Model file for the job. Use its own axes, mm. Give positions to 0.01 mm unless a question says otherwise; leave off trailing zeros. Write each loop counter-clockwise with the first axis right and the second up, starting at its lowest first coordinate (ties: lowest second). Pieces come first, ordered by that corner, then holes. Notation, with made-up numbers: (53.25, 15.25) - (98.25, 15.25) arc R26 ccw to (98.25, 29.25) - close; hole circle Ø11 at (74, -7.5). An arc over 180 degrees is marked (long way). Use a Markdown table: item, result. Add a question column.
```python
from build123d import *

# Parameters (mm, degrees)
SKETCH1_R           = 2.5
BOSS_EXTRUDE1_DEPTH = 10
FILLET1_R           = 20
FILLET2_R           = 2


with BuildPart() as part:
    # Sketch1 → Boss-Extrude1 (new body)
    with BuildSketch(Plane(origin=(0, 0, 0), x_dir=(1, 0, 0), z_dir=(0, 1, 0))):
        with BuildLine():
            Line((0, 0), (0, 125))
            Line((0, 125), (-12.5, 155))
            Line((-12.5, 155), (-25, 125))
            Line((-25, 125), (-38.474856438, 113.744856999))
            ThreePointArc((-38.474856438, 113.744856999), (-43.483141428, 102.313155182), (-37.378629761, 91.427308304))
            Line((-37.378629761, 91.427308304), (-25, 83))
            Line((-25, 83), (-25, 25))
            Line((-25, 25), (-35, 25))
            Line((-35, 25), (-35, 73))
            ThreePointArc((-35, 73), (-37.928932188, 80.071067812), (-45, 83))
            Line((-45, 83), (-45, 58))
            ThreePointArc((-45, 58), (-57.043096437, 48.210936871), (-64.16515139, 62))
            Line((-64.16515139, 62), (-55, 83))
            Line((-55, 83), (-55, 125))
            Line((-55, 125), (-67.5, 155))
            Line((-67.5, 155), (-80, 125))
            Line((-80, 125), (-93.474856438, 113.744856999))
            ThreePointArc((-93.474856438, 113.744856999), (-98.483141428, 102.313155182), (-92.378629761, 91.427308304))
            Line((-92.378629761, 91.427308304), (-80, 83))
            Line((-80, 83), (-80, 25))
            Line((-80, 25), (-90, 25))
            Line((-90, 25), (-90, 73))
            ThreePointArc((-90, 73), (-92.928932188, 80.071067812), (-100, 83))
            Line((-100, 83), (-100, 58))
            ThreePointArc((-100, 58), (-112.043096437, 48.210936871), (-119.16515139, 62))
            Line((-119.16515139, 62), (-110, 83))
            Line((-110, 83), (-110, 125))
            Line((-110, 125), (-122.5, 155))
            Line((-122.5, 155), (-135, 125))
            Line((-135, 125), (-148.474856438, 113.744856999))
            ThreePointArc((-148.474856438, 113.744856999), (-153.483141428, 102.313155182), (-147.378629761, 91.427308304))
            Line((-147.378629761, 91.427308304), (-135, 83))
            Line((-135, 83), (-135, 25))
            Line((-135, 25), (-145, 25))
            Line((-145, 25), (-145, 73))
            ThreePointArc((-145, 73), (-147.928932188, 80.071067812), (-155, 83))
            Line((-155, 83), (-155, 58))
            ThreePointArc((-155, 58), (-167.043096437, 48.210936871), (-174.16515139, 62))
            Line((-174.16515139, 62), (-165, 83))
            Line((-165, 83), (-165, 125))
            Line((-165, 125), (-177.5, 155))
            Line((-177.5, 155), (-190, 125))
            Line((-190, 125), (-203.474856438, 113.744856999))
            ThreePointArc((-203.474856438, 113.744856999), (-208.483141428, 102.313155182), (-202.378629761, 91.427308304))
            Line((-202.378629761, 91.427308304), (-190, 83))
            Line((-190, 83), (-190, 25))
            Line((-190, 25), (-200, 25))
            Line((-200, 25), (-200, 73))
            ThreePointArc((-200, 73), (-202.928932188, 80.071067812), (-210, 83))
            Line((-210, 83), (-210, 58))
            ThreePointArc((-210, 58), (-222.043096437, 48.210936871), (-229.16515139, 62))
            Line((-229.16515139, 62), (-220, 83))
            Line((-220, 83), (-220, 125))
            Line((-220, 125), (-232.5, 155))
            Line((-232.5, 155), (-245, 125))
            Line((-245, 125), (-258.474856438, 113.744856999))
            ThreePointArc((-258.474856438, 113.744856999), (-263.483141428, 102.313155182), (-257.378629761, 91.427308304))
            Line((-257.378629761, 91.427308304), (-245, 83))
            Line((-245, 83), (-245, 25))
            Line((-245, 25), (-255, 25))
            Line((-255, 25), (-255, 73))
            ThreePointArc((-255, 73), (-257.928932188, 80.071067812), (-265, 83))
            Line((-265, 83), (-265, 58))
            ThreePointArc((-265, 58), (-277.043096437, 48.210936871), (-284.16515139, 62))
            Line((-284.16515139, 62), (-275, 83))
            Line((-275, 83), (-275, 125))
            Line((-275, 125), (-287.5, 155))
            Line((-287.5, 155), (-300, 125))
            Line((-300, 125), (-300, 0))
            Line((-300, 0), (0, 0))
        make_face()
        with Locations(Location((-12.5, 125, 0), (0, 0, 270))):
            Circle(SKETCH1_R, mode=Mode.SUBTRACT)
        with Locations(Location((-64, 89, 0), (0, 0, 270))):
            Circle(SKETCH1_R, mode=Mode.SUBTRACT)
        with Locations(Location((-67.5, 125, 0), (0, 0, 270))):
            Circle(SKETCH1_R, mode=Mode.SUBTRACT)
        with Locations(Location((-119, 89, 0), (0, 0, 270))):
            Circle(SKETCH1_R, mode=Mode.SUBTRACT)
        with Locations(Location((-122.5, 125, 0), (0, 0, 270))):
            Circle(SKETCH1_R, mode=Mode.SUBTRACT)
        with Locations(Location((-174, 89, 0), (0, 0, 270))):
            Circle(SKETCH1_R, mode=Mode.SUBTRACT)
        with Locations(Location((-177.5, 125, 0), (0, 0, 270))):
            Circle(SKETCH1_R, mode=Mode.SUBTRACT)
        with Locations(Location((-229, 89, 0), (0, 0, 270))):
            Circle(SKETCH1_R, mode=Mode.SUBTRACT)
        with Locations(Location((-232.5, 125, 0), (0, 0, 270))):
            Circle(SKETCH1_R, mode=Mode.SUBTRACT)
        with Locations(Location((-284, 89, 0), (0, 0, 270))):
            Circle(SKETCH1_R, mode=Mode.SUBTRACT)
    extrude(amount=BOSS_EXTRUDE1_DEPTH)

    # Fillet1
    fillet1_edges = [part.edges().sort_by_distance(p)[0] for p in [
        (-300, 5, -125),
        (-275, 5, -125),
        (-275, 5, -83),
        (-245, 5, -83),
        (-245, 5, -125),
        (-220, 5, -125),
        (-220, 5, -83),
        (-190, 5, -83),
        (-190, 5, -125),
        (-165, 5, -125),
        (-165, 5, -83),
        (-135, 5, -83),
        (-135, 5, -125),
        (-110, 5, -125),
        (-110, 5, -83),
        (-80, 5, -83),
        (-80, 5, -125),
        (-55, 5, -125),
        (-55, 5, -83),
        (-25, 5, -83),
        (-25, 5, -125),
        (0, 5, -125),
    ]]
    fillet(fillet1_edges, radius=FILLET1_R)

    # Fillet2
    fillet2_edges = [part.edges().sort_by_distance(p)[0] for p in [
        (-265, 5, -83),
        (-210, 5, -83),
        (-155, 5, -83),
        (-100, 5, -83),
        (-45, 5, -83),
    ]]
    fillet(fillet2_edges, radius=FILLET2_R)


solid = part.part
```
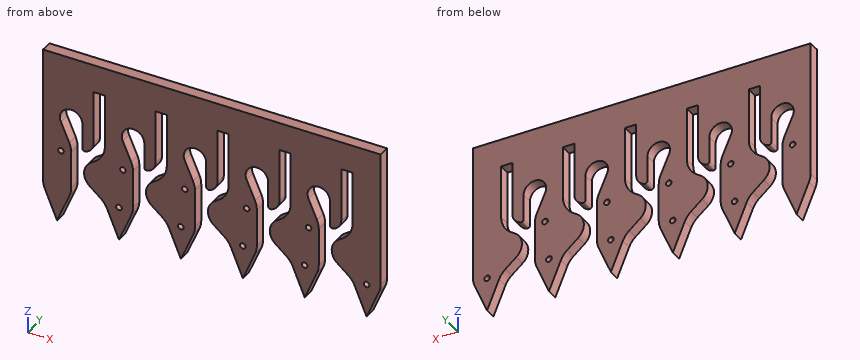
(1) Band-saw the part on B-B (y = 7.25). Give the number of separate pieces and of enclosed holes in the cut face, then the cut area to 3 significant figures.
(2) Flat gauge pins, fed straight in: pin 1 (12 mm diameter, centred on x = -110, z = -58, fed in from +Y); pin 2 (5 mm diameter, centred on x = -139.5, y = 6.5, fed in from -Z); pin 3 (1.5 mm diameter, centred on x = -190.5, y = 5.5, fed in from -Z). Where does each tip first touch, or does it go through?
(3) Probe probe 1 along X at (y, z) = (0.75, -36.5); probe 2 along Z at (x, y) = (-284, 5.75); probe 3 along X at (y, z) = (3, -129). List the from-to ranges inside material, lowest first. Write a range as [from, to].
(4) Band-saw the part on A-A (z = -139). Write the cut outline in (x, y), then the cut area to 3 significant figures.
(5) Band-saw the part on C-C (x = -268). Write the cut outline in (y, z).
Model answer:
| question | item | result |
|---|---|---|
| 1 | separate pieces | 1 |
| 1 | enclosed holes | 10 |
| 1 | area | 30,100 mm^2 |
| 2 | pin 1 | passes through |
| 2 | pin 2 | stops at z = -123.52 |
| 2 | pin 3 | stops at z = -126.4 |
| 3 | probe 1 | x = [-300, -255], [-245, -200], [-190, -145], [-135, -90], [-80, -35], [-25, 0] |
| 3 | probe 2 | z = [-146.6, -91.5], [-86.5, -62.38], [-53.64, 0] |
| 3 | probe 3 | x = [-298.33, -276.67], [-243.34, -221.67], [-188.34, -166.67], [-133.34, -111.67], [-78.34, -56.67], [-23.34, -1.67] |
| 4 | outline | (-294.17, 0) - (-280.83, 0) - (-280.83, 10) - (-294.17, 10) - close; (-239.17, 0) - (-225.83, 0) - (-225.83, 10) - (-239.17, 10) - close; (-184.17, 0) - (-170.83, 0) - (-170.83, 10) - (-184.17, 10) - close; (-129.17, 0) - (-115.83, 0) - (-115.83, 10) - (-129.17, 10) - close; (-74.17, 0) - (-60.83, 0) - (-60.83, 10) - (-74.17, 10) - close; (-19.17, 0) - (-5.83, 0) - (-5.83, 10) - (-19.17, 10) - close |
| 4 | area | 800 mm^2 |
| 5 | outline | (0, -50.86) - (10, -50.86) - (10, 0) - (0, 0) - close |
